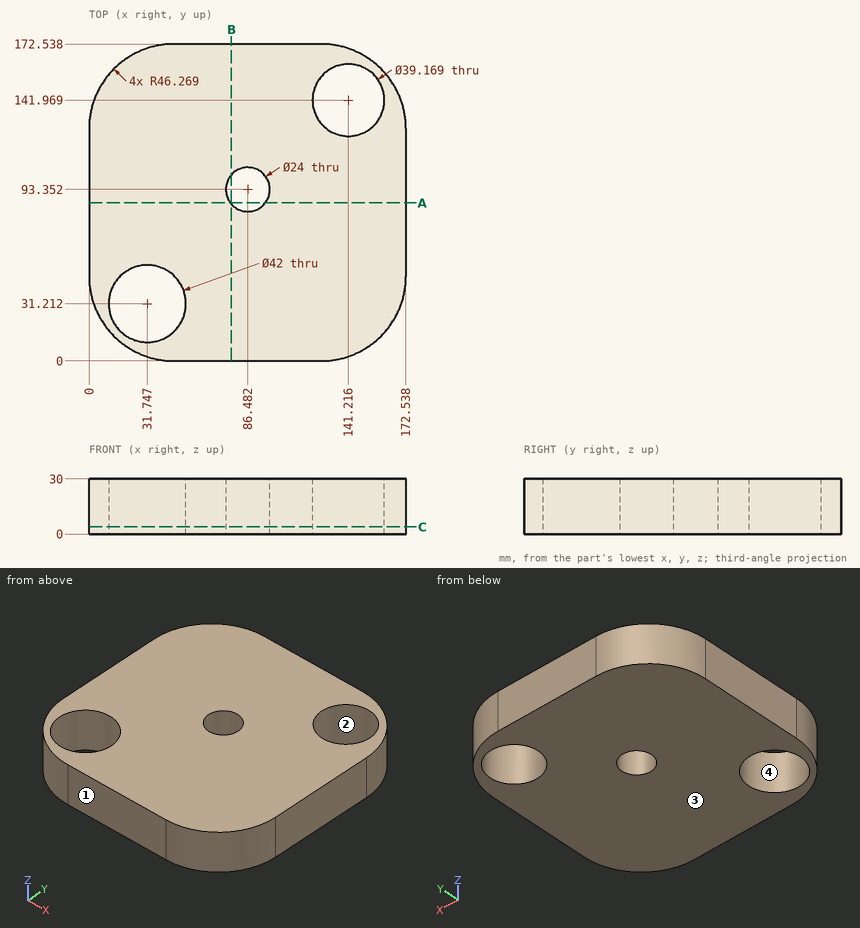
Check sheet for the drawn part. Datum: minimum x, y, z corner. Units: mm. Round coordinates to 2 decimals unless told otherwise and drop trailing zeros. Loops run counter-clockwise (first coordinate to the right, second up) from the corner with the lowest first, then second, coordinate; pieces in that order, holes last. Notation, with made-up numbers: M 67,84.25 L 96,84.25 A32 cw 96,113.25 Z; hole C 73.5,69 d7. An arc over 180 degrees is marked long. Write each question's results on one line, items separated by ' | '.
1) Mould release check, pull along Y, two halves, no side actions. Record for the marked faces 1, 2, 3 and 4: released by +Y, released by -Y, zero draft, split by the parting line, or undercut.
Checks:
face 1: released by -Y | face 2: undercut | face 3: zero draft | face 4: undercut
2) Scan lines: L1, parallel to Y at x = 91, z = 5.75 (1 decimal); L2, parallel to X at y = 85, z = 10.75 (1 decimal); L3, parallel to Y at x = 94.5, z = 27 (1 decimal). Record each from-to range of solid material in increasing order. Write a range as from..to.
Checks:
L1: y = 0..82.2, 104.5..172.5 | L2: x = 0..77.9, 95.1..172.5 | L3: y = 0..84.4, 102.3..172.5
3) Section check A-A on y = 86. Record the boundary of the cut face in (x, z) (1 decimal), then the cut area to 3 significant figures.
Checks:
outline: M 0,0 L 77,0 L 77,30 L 0,30 Z; M 96,0 L 172.5,0 L 172.5,30 L 96,30 Z | area: 4,610 mm2
4) Gauge pin test, flat ends, axial feed: P1, Ø1.5, axis at y = 141, z = 20.5, coming from the -X side; P2, Ø14.5, axis at x = 86.48, y = 93.35, coming from the +Z side; P3, Ø4, axis at y = 133.5, z = 26, coming from the +X side. Record the tip position at first contact, or that the pin passes through.
Checks:
P1: stops at x = 2.16 | P2: passes through | P3: stops at x = 172.24
5) Section check C-C on z = 4. Record the boundary of the cut face in (x, y) (1 decimal), then the cut area to 3 significant figures.
Checks:
outline: M 0,46.3 A46.3 ccw 46.3,0 L 126.3,0 A46.3 ccw 172.5,46.3 L 172.5,126.3 A46.3 ccw 126.3,172.5 L 46.3,172.5 A46.3 ccw 0,126.3 Z; hole C 31.7,31.2 d42; hole C 86.5,93.4 d24; hole C 141.2,142 d39.2 | area: 24,900 mm2
6) Section check B-B on x = 77.5. Record the boundary of the cut face in (y, z) (1 decimal).
Checks:
outline: M 0,0 L 85.4,0 L 85.4,30 L 0,30 Z; M 101.3,0 L 172.5,0 L 172.5,30 L 101.3,30 Z
